Could you check a few things on this model? Use its own coordinates, in mm. A direction names the side the tool comes from. Give positions to 0.01 mm unless a question says otherwise; leave off trailing zeros. Write each loop counter-clockwise with the first axis right and the second up, starting at its lowest first coordinate (ties: lowest second). Pieces come first, ordered by that corner, then holes. Notation, with made-up numbers: M 30,11 L 48,11 A33 ccw 48,44 Z; hole C -7.5,-8.5 d11. An arc over 180 degrees is marked long. Use one line per item in the form item = value.
from build123d import *

# Parameters (mm, degrees)
F1_DEPTH = 8


with BuildPart() as f1:
    # F0 (on Top) → F1 (new body)
    with BuildSketch(Plane.XY):
        with BuildLine():
            Line((8, 0), (0, 0))
            Line((0, 0), (0, -6))
            Line((0, -6), (5.606788, -6))
            ThreePointArc((5.606788, -6), (7.229002, -6.597785), (8.075428, -8.105263))
            ThreePointArc((8.075428, -8.105263), (13.599168, -13.860919), (20.926175, -10.705882))
            ThreePointArc((20.926175, -10.705882), (21.471115, -10.188288), (22.198722, -10))
            Line((22.198722, -10), (25.312175, -10))
            ThreePointArc((25.312175, -10), (26.019282, -9.707107), (26.312175, -9))
            ThreePointArc((26.312175, -9), (26.019282, -8.292893), (25.312175, -8))
            Line((25.312175, -8), (21.915823, -8))
            Line((21.915823, -8), (20.98762, -8))
            ThreePointArc((20.98762, -8), (20.155569, -8.251925), (19.603004, -8.923077))
            ThreePointArc((19.603004, -8.923077), (9.98762, -7), (19.603004, -5.076923))
            ThreePointArc((19.603004, -5.076923), (20.155569, -5.748075), (20.98762, -6))
            Line((20.98762, -6), (21.915823, -6))
            Line((21.915823, -6), (25.312175, -6))
            ThreePointArc((25.312175, -6), (26.019282, -5.707107), (26.312175, -5))
            ThreePointArc((26.312175, -5), (26.019282, -4.292893), (25.312175, -4))
            Line((25.312175, -4), (22.198722, -4))
            ThreePointArc((22.198722, -4), (21.471115, -3.811712), (20.926175, -3.294118))
            ThreePointArc((20.926175, -3.294118), (18.383118, -0.878678), (14.98762, 0))
            Line((14.98762, 0), (8, 0))
        make_face()
    extrude(amount=F1_DEPTH)


solid = f1.part
1) I want a section at B-B, the plane x = 17.25. Please give me the cut outline in (y, z), plus the area to 3 significant figures.
Checked values:
outline = M -13.62,0 L -11.46,0 L -11.46,8 L -13.62,8 Z; M -2.54,0 L -0.38,0 L -0.38,8 L -2.54,8 Z
area = 34.6 mm2
2) I want a section at C-C, the plane z = 5.5. Please give me the cut outline in (x, y), plus the area to 3 significant figures.
Checked values:
outline = M 0,-6 L 5.61,-6 A2.5 cw 8.08,-8.11 A7 ccw 20.93,-10.71 A1.5 cw 22.2,-10 L 25.31,-10 A1 ccw 26.31,-9 A1 ccw 25.31,-8 L 20.99,-8 A1.5 ccw 19.6,-8.92 A5 cw long 19.6,-5.08 A1.5 ccw 20.99,-6 L 25.31,-6 A1 ccw 26.31,-5 A1 ccw 25.31,-4 L 22.2,-4 A1.5 cw 20.93,-3.29 A7 ccw 14.99,0 L 0,0 Z
area = 148 mm2
3) Thinking about a two-plate mould opening in X: for faces 1 (the cylindrical face through (18.426, -0.903, 3.944)), 2 (the cylindrical face through (20.166, -8.245, 3.944)), 3 (the flat face through (24, -10, 4)), 4 (the flat face through (0, -3, 4)), which applies, released by +X, released by -X, zero draft, split by the parting line, or undercut?
Checked values:
face_1 = released by +X
face_2 = undercut
face_3 = zero draft
face_4 = released by -X
4) I want a section at A-A, the plane y = -11.5. Please give me the cut outline in (x, z), plus the area to 3 significant figures.
Checked values:
outline = M 9.63,0 L 12.81,0 L 12.81,8 L 9.63,8 Z; M 17.17,0 L 20.35,0 L 20.35,8 L 17.17,8 Z
area = 50.9 mm2
5) I want a section at D-D, the plane y = -7. Please give me the cut outline in (x, z).
Checked values:
outline = M 7.61,0 L 9.99,0 L 9.99,8 L 7.61,8 Z
6) For faces 5 (the flat face through (3, -6, 4)), 6 (the flat face through (23, -8, 4)), 7 (the flat face through (24, -4, 4)), which set-ups out of +Z, -Z, +X, -X, +Y, -Y let a thin tool reach every point of the face, with its end or its side?
Checked values:
face_5 = +Z, -Z, -X, -Y
face_6 = +Z, -Z, +X
face_7 = +Z, -Z, +X, +Y
7) If I drill on L1, parallel to Y at x = 22.5, z = 2; L2, parallel to Y at x = 15.25, z = 3; L3, parallel to X at y = -3, z = 3.5, over which ranges is the centre line in solid material (lowest first)?
Checked values:
L1 = -10 to -8, -6 to -4
L2 = -14 to -11.99, -2.01 to 0
L3 = 0 to 11.99, 17.99 to 20.73
8) For pin 1 Ø0.9 at (x, z) = (24, 3) entering from -Y; pin 2 Ø1.7 at (x, z) = (3.5, 2.5) entering from -Y; pin 3 Ø3.5 at (x, z) = (22.5, 3.5) entering from -Y; pin 4 Ø5 at (x, y) = (4, -9) entering from +Z, each with a flat end and sliding along its axis, tell me the tip position at first contact or that it passes through.
Checked values:
pin_1 = -10
pin_2 = -6
pin_3 = -10.97
pin_4 = through
